Verification items for the finished model (mm, model axes). Face numbers are marked on the shaded views. Give positions to 0.01 mm unless a question says otherwise; leave off trailing zeros. Write each loop counter-clockwise with the first axis right and the second up, starting at its lowest first coordinate (ties: lowest second). Pieces come first, ordered by that corner, then holes.
from build123d import *

# Parameters (mm, degrees)
F0_R     = 25
F0_R_2   = 23.5
F1_DEPTH = 100
F2_R     = 25
F3_DEPTH = 5
F4_R     = 1
F5_R     = 0.5
F6_DEPTH = 25


with BuildPart() as f1:
    # F0 (on Top) → F1 (new body)
    with BuildSketch(Plane.XY):
        Circle(F0_R)
        Circle(F0_R_2, mode=Mode.SUBTRACT)
    extrude(amount=F1_DEPTH)

    # F2 (on Top) → F3 (join)
    with BuildSketch(Plane.XY):
        Circle(F2_R)
    extrude(amount=-F3_DEPTH)

    # F4
    f4_edges = [f1.edges().sort_by_distance(p)[0] for p in [
        (-25, 0, -5),
        (-25, 0, 100),
    ]]
    fillet(f4_edges, radius=F4_R)

    # F5 (on Top) → F6 (cut)
    with BuildSketch(Plane.XY):
        Circle(F5_R)
    extrude(amount=-F6_DEPTH, mode=Mode.SUBTRACT)


solid = f1.part
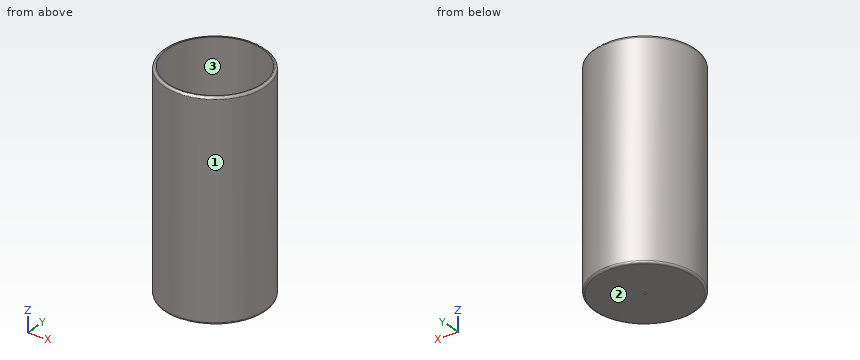
Item 1: Depth check by flat-ended pin: pin 1 (6 mm diameter, centred on x = -2, z = 71.5, fed in from +Y); pin 2 (6 mm diameter, centred on y = 20, z = 52.5, fed in from +X); pin 3 (1.5 mm diameter, centred on y = 9, z = 19.5, fed in from +X); pin 4 (12 mm diameter, centred on y = -5, z = 86, fed in from +X). Enter the tip coordinate at first touch or a pass-through.
Answer key:
pin 1: stops at y = 25
pin 2: stops at x = 18.33
pin 3: stops at x = 23.6
pin 4: stops at x = 25
Item 2: Scan lines: line 1 along Y through (x, z) = (0, -3.6); line 2 along Y through (x, z) = (0, 20); line 3 along Z through (x, y) = (11, 19). Record each from-to range of solid material in increasing order.
Answer key:
line 1: y = -25 to -0.5, 0.5 to 25
line 2: y = -25 to -23.5, 23.5 to 25
line 3: z = -5 to 0
Item 3: Sectioned sample at A-A on z = 91.5. Record the cut outline in (x, y).
Answer key:
outline: circle Ø50 at (0, 0); hole circle Ø47 at (0, 0)
Item 4: Release check for a two-part mould opening along X. For the marked faces 1, 2 and 3 record: released by +X, released by -X, zero draft, split by the parting line, or undercut.
Answer key:
face 1: split by the parting line
face 2: zero draft
face 3: undercut
